Source: CAD feature listing. Evaluate the final solid. Frame: model axes, mm. Face numbers are marked on the shaded views. A direction names the side the tool comes from. Give positions to 0.01 mm unless a question says otherwise; leave off trailing zeros. Loops run counter-clockwise (first coordinate to the right, second up) from the corner with the lowest first, then second, coordinate; pieces in that order, holes last.
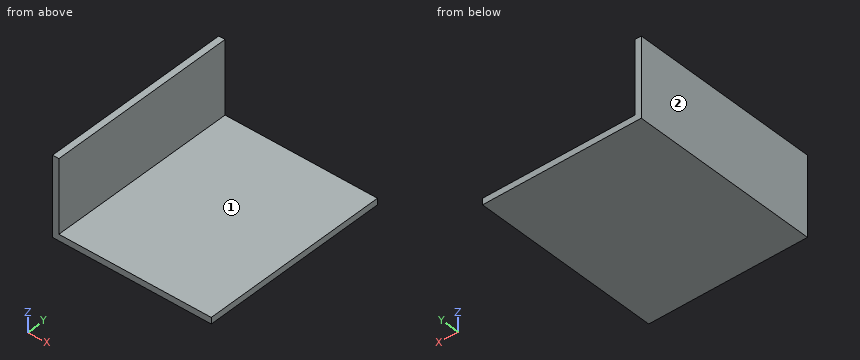
from build123d import *

# Parameters (mm, degrees)
SKETCH_1_W          = 200
SKETCH_1_H          = 240
SKETCH_1_R          = 13
EXTRUDE_393_DEPTH   = 8
SKETCH_2_W          = 8
SKETCH_2_H          = 240
EXTRUDE_1_DEPTH     = 92
SKETCH_3_R          = 13
CUT_EXTRUDE_1_DEPTH = 329.024389337
SKETCH_5_W          = 192
SKETCH_5_H          = 240
EXTRUDE_2_DEPTH     = 8
SKETCH_6_W          = 92
SKETCH_6_H          = 240
EXTRUDE_3_DEPTH     = 8


with BuildPart() as part:
    # 草图1 → Extrude 393 (new body)
    with BuildSketch(Plane.XY):
        with Locations((100, 120)):
            Rectangle(SKETCH_1_W, SKETCH_1_H)
        with Locations((160, 40)):
            Circle(SKETCH_1_R, mode=Mode.SUBTRACT)
        with Locations((160, 120)):
            Circle(SKETCH_1_R, mode=Mode.SUBTRACT)
        with Locations((160, 200)):
            Circle(SKETCH_1_R, mode=Mode.SUBTRACT)
    extrude(amount=EXTRUDE_393_DEPTH)

    # 草图2 → 凸台-拉伸1 (add)
    with BuildSketch(Plane.XY.offset(8)):
        with Locations((4, 120)):
            Rectangle(SKETCH_2_W, SKETCH_2_H)
    extrude(amount=EXTRUDE_1_DEPTH)

    # 草图3 → 切除-拉伸1 (cut, through all)
    with BuildSketch(Plane.ZY):
        with Locations((52, 200)):
            Circle(SKETCH_3_R)
        with Locations((52, 120)):
            Circle(SKETCH_3_R)
        with Locations((52, 40)):
            Circle(SKETCH_3_R)
    extrude(amount=-CUT_EXTRUDE_1_DEPTH, mode=Mode.SUBTRACT)

    # 草图5 → 凸台-拉伸2 (add)
    with BuildSketch(Plane.XY.offset(8)):
        with Locations((104, 120)):
            Rectangle(SKETCH_5_W, SKETCH_5_H)
    extrude(amount=-EXTRUDE_2_DEPTH)

    # 草图6 → 凸台-拉伸3 (add)
    with BuildSketch(Plane(origin=(8, 0, 0), x_dir=(0, 0, -1), z_dir=(1, 0, 0))):
        with Locations((-54, 120)):
            Rectangle(SKETCH_6_W, SKETCH_6_H)
    extrude(amount=-EXTRUDE_3_DEPTH)


solid = part.part
1) Cut plane A-A (y = 211). Return loops of the section in (x, z), and give its area (3 significant figures).
Checks:
outline: (0, 0) - (200, 0) - (200, 8) - (8, 8) - (8, 100) - (0, 100) - close
area: 2,340 mm2
2) Cut plane C-C (x = 84). Return loops of the section in (y, z), and give its area (3 significant figures).
Checks:
outline: (0, 0) - (240, 0) - (240, 8) - (0, 8) - close
area: 1,920 mm2
3) Contact query for flat-ended pins moving along their axis: P1, Ø2, axis at y = 185.5, z = 43.5, coming from the +X side; P2, Ø8, axis at x = 37, y = 68.5, coming from the +Z side. Output: stop coordinate, or through.
Checks:
P1: stops at x = 8
P2: stops at z = 8
4) Ray query, probe 1 along Z at (x, y) = (9, 76.5). Return the intervals inside material, ascending.
Checks:
probe 1: z = 0 to 8
5) Cut plane B-B (z = 41). Return loops of the section in (x, y), and give its area (3 significant figures).
Checks:
outline: (0, 0) - (8, 0) - (8, 240) - (0, 240) - close
area: 1,920 mm2
6) Reachability of the marked faces 1 and 2 from +Z, -Z, +X, -X, +Y, -Y: full face, straight path, thin tool, end or side. Return the list, or none.
Checks:
face 1: +Z, +X, +Y, -Y
face 2: +Z, -Z, -X, +Y, -Y
